from build123d import *

# Parameters (mm, degrees)
SKETCH1_R           = 2.55
BOSS_EXTRUDE2_DEPTH = 10
SKETCH2_R           = 2.55
BOSS_EXTRUDE3_DEPTH = 2
SKETCH3_W           = 30
SKETCH3_H           = 2
CUT_EXTRUDE1_DEPTH  = 35
SKETCH4_W           = 19.809531665
SKETCH4_H           = 16
CUT_EXTRUDE2_DEPTH  = 19
FILLET1_R           = 10


with BuildPart() as part:
    # Sketch1 → Boss-Extrude2 (new body)
    with BuildSketch(Plane.XY):
        with BuildLine():
            ThreePointArc((18.024150889, 186.79103775), (10.644862344, 190.724335457), (2.347067513, 191.759386777))
            ThreePointArc((2.347067513, 191.759386777), (0, 191.690468331), (-2.347067513, 191.759386777))
            ThreePointArc((-2.347067513, 191.759386777), (-10.644862344, 190.724335457), (-18.024150889, 186.79103775))
            ThreePointArc((-18.024150889, 186.79103775), (-28.284271247, 194.215728749), (-35.708962247, 204.475849108))
            ThreePointArc((-35.708962247, 204.475849108), (-31.77566454, 211.855137653), (-30.74061322, 220.152932484))
            ThreePointArc((-30.74061322, 220.152932484), (-30.809531665, 222.499999997), (-30.74061322, 224.84706751))
            ThreePointArc((-30.74061322, 224.84706751), (-31.77566454, 233.14486234), (-35.708962247, 240.524150885))
            ThreePointArc((-35.708962247, 240.524150885), (-28.284271247, 250.784271244), (-18.024150889, 258.208962244))
            ThreePointArc((-18.024150889, 258.208962244), (-10.644862344, 254.275664537), (-2.347067513, 253.240613217))
            ThreePointArc((-2.347067513, 253.240613217), (0, 253.309531662), (2.347067513, 253.240613217))
            ThreePointArc((2.347067513, 253.240613217), (10.644862344, 254.275664537), (18.024150889, 258.208962244))
            ThreePointArc((18.024150889, 258.208962244), (28.284271247, 250.784271244), (35.708962247, 240.524150885))
            ThreePointArc((35.708962247, 240.524150885), (31.77566454, 233.14486234), (30.74061322, 224.84706751))
            ThreePointArc((30.74061322, 224.84706751), (30.809531665, 222.499999997), (30.74061322, 220.152932484))
            ThreePointArc((30.74061322, 220.152932484), (31.77566454, 211.855137653), (35.708962247, 204.475849108))
            ThreePointArc((35.708962247, 204.475849108), (28.284271247, 194.215728749), (18.024150889, 186.79103775))
        make_face()
        with Locations((-22.627416998, 245.127416995)):
            Circle(SKETCH1_R, mode=Mode.SUBTRACT)
        with Locations((-22.627416998, 199.872582999)):
            Circle(SKETCH1_R, mode=Mode.SUBTRACT)
        with Locations((22.627416998, 199.872582999)):
            Circle(SKETCH1_R, mode=Mode.SUBTRACT)
        with Locations((22.627416998, 245.127416995)):
            Circle(SKETCH1_R, mode=Mode.SUBTRACT)
        with BuildLine():
            Line((-15, 218.499999997), (-15, 199.25))
            Line((-15, 199.25), (15, 199.25))
            Line((15, 199.25), (15, 218.499999997))
            ThreePointArc((15, 218.499999997), (19, 222.499999997), (15, 226.499999997))
            Line((15, 226.499999997), (15, 245.749999994))
            Line((15, 245.749999994), (-15, 245.749999994))
            Line((-15, 245.749999994), (-15, 226.499999997))
            ThreePointArc((-15, 226.499999997), (-19, 222.499999997), (-15, 218.499999997))
        make_face(mode=Mode.SUBTRACT)
    extrude(amount=BOSS_EXTRUDE2_DEPTH)

    # Sketch2 → Boss-Extrude3 (add)
    with BuildSketch(Plane.XY.offset(10)):
        with BuildLine():
            ThreePointArc((18.024150889, 186.79103775), (28.284271247, 194.215728749), (35.708962247, 204.475849108))
            ThreePointArc((35.708962247, 204.475849108), (31.77566454, 211.855137653), (30.74061322, 220.152932484))
            ThreePointArc((30.74061322, 220.152932484), (30.809531665, 222.499999997), (30.74061322, 224.84706751))
            ThreePointArc((30.74061322, 224.84706751), (31.77566454, 233.14486234), (35.708962247, 240.524150885))
            ThreePointArc((35.708962247, 240.524150885), (28.284271247, 250.784271244), (18.024150889, 258.208962244))
            ThreePointArc((18.024150889, 258.208962244), (10.644862344, 254.275664537), (2.347067513, 253.240613217))
            ThreePointArc((2.347067513, 253.240613217), (0, 253.309531662), (-2.347067513, 253.240613217))
            ThreePointArc((-2.347067513, 253.240613217), (-10.644862344, 254.275664537), (-18.024150889, 258.208962244))
            ThreePointArc((-18.024150889, 258.208962244), (-28.284271247, 250.784271244), (-35.708962247, 240.524150885))
            ThreePointArc((-35.708962247, 240.524150885), (-31.77566454, 233.14486234), (-30.74061322, 224.84706751))
            ThreePointArc((-30.74061322, 224.84706751), (-30.809531665, 222.499999997), (-30.74061322, 220.152932484))
            ThreePointArc((-30.74061322, 220.152932484), (-31.77566454, 211.855137653), (-35.708962247, 204.475849108))
            ThreePointArc((-35.708962247, 204.475849108), (-28.284271247, 194.215728749), (-18.024150889, 186.79103775))
            ThreePointArc((-18.024150889, 186.79103775), (-10.644862344, 190.724335457), (-2.347067513, 191.759386777))
            ThreePointArc((-2.347067513, 191.759386777), (0, 191.690468331), (2.347067513, 191.759386777))
            ThreePointArc((2.347067513, 191.759386777), (10.644862344, 190.724335457), (18.024150889, 186.79103775))
        make_face()
        with Locations((-22.627416998, 245.127416995)):
            Circle(SKETCH2_R, mode=Mode.SUBTRACT)
        with Locations((-22.627416998, 199.872582999)):
            Circle(SKETCH2_R, mode=Mode.SUBTRACT)
        with Locations((22.627416998, 199.872582999)):
            Circle(SKETCH2_R, mode=Mode.SUBTRACT)
        with Locations((22.627416998, 245.127416995)):
            Circle(SKETCH2_R, mode=Mode.SUBTRACT)
        with BuildLine():
            Line((-15, 245.749999994), (-15, 226.499999997))
            ThreePointArc((-15, 226.499999997), (-19, 222.499999997), (-15, 218.499999997))
            Line((-15, 218.499999997), (15, 218.499999997))
            ThreePointArc((15, 218.499999997), (19, 222.499999997), (15, 226.499999997))
            Line((15, 226.499999997), (15, 245.749999994))
            Line((15, 245.749999994), (-15, 245.749999994))
        make_face(mode=Mode.SUBTRACT)
    extrude(amount=BOSS_EXTRUDE3_DEPTH)

    # Sketch3 → Cut-Extrude1 (cut)
    with BuildSketch(Plane.XY.offset(12)):
        with Locations((0, 246.749999994)):
            Rectangle(SKETCH3_W, SKETCH3_H)
    extrude(amount=-CUT_EXTRUDE1_DEPTH, mode=Mode.SUBTRACT)

    # Sketch4 → Cut-Extrude2 (cut)
    with BuildSketch(Plane(origin=(0, 0, 0), x_dir=(-1, 0, 0), z_dir=(0, 0, -1))):
        with Locations((24.904765833, 222.499999997)):
            Rectangle(SKETCH4_W, SKETCH4_H)
    extrude(amount=-CUT_EXTRUDE2_DEPTH, mode=Mode.SUBTRACT)

    # Fillet1
    # the kernel refuses this fillet: 10 mm, written as the material it takes off along each edge
    with BuildSketch(Plane(origin=(-15, 218.499999997, -10), x_dir=(0, -1, 0), z_dir=(0, 0, 1))) as fillet1_piece_1:
        with BuildLine():
            CenterArc((10, 8), FILLET1_R, 180, 53.130102354)
            Line((0, 8), (-0.2, 8))
            Line((-0.2, 8), (-0.2, 0))
            Line((-0.2, 0), (0, -0.2))
            ThreePointArc((0, -0.2), (2, -0.2), (3.88, -0.16))
            Line((3.88, -0.16), (4, 0))
        make_face()
    extrude(amount=42, mode=Mode.SUBTRACT)


solid = part.part
CAD build for the part. Positions are in the model's coordinates, mm. A direction names the side the tool comes from. Give positions to 0.01 mm unless a question says otherwise; leave off trailing zeros. Loops run counter-clockwise (first coordinate to the right, second up) from the corner with the lowest first, then second, coordinate; pieces in that order, holes last. Notation, with made-up numbers: M 67.5,-12.75 L 119.5,-12.75 A18 cw 119.5,-4.75 Z; hole C 1.25,3 d5. An arc over 180 degrees is marked long. Answer in a Markdown table with one row per item. Add a question column.
Item 1: Drop flat-ended pins along their axis: P1, Ø4, axis at x = 4, z = 10.5, coming from the +Y side; P2, Ø4, axis at x = -14, z = 8, coming from the +Y side; P3, Ø6, axis at x = 9, z = 1.5, coming from the -Y side. Give the stop position or say it passes through.
Item 2: Band-saw the part on D-D on y = 234.5. Give the cut face in (x, z), then the cut area to 3 significant figures.
Item 3: Mould opens along X. For faces 5 (the face through (28.41, 250.66, 5.92)), 6 (the face through (19, 222.4, 5.9)), 7 (the face through (0, 199.25, 5)) say: +X half, -X half, draft (parallel to the pull), parting line (faces both ways), or undercut.
Item 4: Probe probe 1 along X at (y, z) = (246, 6.75); probe 2 along Y at (x, z) = (-2, 8); probe 3 along Y at (x, z) = (22, 7.75). List the from-to ranges inside material, lowest first.
Item 5: Tool access for faces 1 (the face through (-15, 207, 5)), 2 (the face through (-23, 230.5, 6)), 3 (the face through (16, 215, 0)), 4 (the face through (-15, 239, 6)): list every direction of +Z, -Z, +X, -X, +Y, -Y with a clear straight run to the whole face (end or side of a thin tool).
Item 6: Band-saw the part on A-A on x = 6. Give the cut face in (y, z).
Item 7: Band-saw the part on C-C on y = 243.5. Give the cut face in (x, z).
Item 8: Band-saw the part on B-B on z = 8.25. Give the cut face in (x, y).
Reply:
| question | item | result |
|---|---|---|
| 1 | P1 | stops at y = 253.32 |
| 1 | P2 | stops at y = 256.77 |
| 1 | P3 | stops at y = 190.25 |
| 2 | outline | M -32.25,0 L -15,0 L -15,12 L -32.25,12 Z; M 15,0 L 32.25,0 L 32.25,12 L 15,12 Z |
| 2 | area | 414 mm^2 |
| 3 | face 5 | +X half |
| 3 | face 6 | -X half |
| 3 | face 7 | undercut |
| 4 | probe 1 | x = -32.37 to -25.02, -20.23 to -15, 15 to 20.23, 25.02 to 32.37 |
| 4 | probe 2 | y = 191.74 to 199.25, 247.75 to 253.26 |
| 4 | probe 3 | y = 189.09 to 197.4, 202.34 to 242.66, 247.6 to 255.91 |
| 5 | face 1 | -Z |
| 5 | face 2 | +Z, -Z, -X |
| 5 | face 3 | -Z, +X, -X, +Y, -Y |
| 5 | face 4 | +Z, -Z |
| 6 | outline | M 191.68,0 L 199.25,0 L 199.25,10 L 218.5,10 L 218.5,12 L 191.68,12 Z; M 247.75,0 L 253.32,0 L 253.32,12 L 247.75,12 Z |
| 7 | outline | M -34.04,0 L -24.59,0 L -24.59,12 L -34.04,12 Z; M -20.66,0 L -15,0 L -15,12 L -20.66,12 Z; M 15,0 L 20.66,0 L 20.66,12 L 15,12 Z; M 24.59,0 L 34.04,0 L 34.04,12 L 24.59,12 Z |
| 8 | outline | M -35.71,204.48 A40 ccw -18.02,186.79 A23 cw -2.35,191.76 A40 ccw 2.35,191.76 A23 cw 18.02,186.79 A40 ccw 35.71,204.48 A23 cw 30.74,220.15 A40 ccw 30.74,224.85 A23 cw 35.71,240.52 A40 ccw 18.02,258.21 A23 cw 2.35,253.24 A40 ccw -2.35,253.24 A23 cw -18.02,258.21 A40 ccw -35.71,240.52 A23 cw -31.11,230.5 L -15,230.5 L -15,247.75 L 15,247.75 L 15,226.5 A4 cw 15,218.5 L 15,199.25 L -15,199.25 L -15,214.5 L -31.11,214.5 A23 cw Z; hole C -22.63,199.87 d5.1; hole C -22.63,245.13 d5.1; hole C 22.63,199.87 d5.1; hole C 22.63,245.13 d5.1 |
